Design review of the part built by this model. Coordinates are the model's own, in mm. Face numbers are marked on the shaded views. A direction names the side the tool comes from. Coordinates: 2 decimals unless noted, no trailing zeros. Write each loop counter-clockwise with the first axis right and the second up, starting at its lowest first coordinate (ties: lowest second). Pieces come first, ordered by that corner, then holes.
Q1. To check wall thickness, follow probe 1 along X at (y, z) = (6.25, 5); probe 2 along Z at (x, y) = (16.75, 2); probe 3 along Z at (x, y) = (1.25, 25). State the ranges of each line that lie inside material, in increasing order.
Q2. Add section D-D, the plane z = 59. Give the boundary of the cut face in (x, y).
Q3. Add section A-A, the plane y = 7. Give the boundary of the cut face in (x, z), plus the area to 3 significant figures.
Q4. Clearance check with flat-ended pins moving along their axes: pin 1 Ø2.5 at (x, z) = (5, 65) entering from -Y; pin 2 Ø10 at (x, z) = (9, 39) entering from -Y; pin 3 Ø6 at (x, z) = (13.5, 38.5) entering from +Y. State where each tip first meets the part, or that it passes through.
Q5. Add section C-C, the plane y = 16.5. Give the boundary of the cut face in (x, z).
Q6. Machinability: for the marked faces 1, 2 and 3, which of the approach directions +Z, -Z, +X, -X, +Y, -Y give a long, thin tool a straight path to every point of the face, cutting with its end or side? Answer none if there is none.
Q7. Add section B-B, the plane x = 9.25. Give the boundary of the cut face in (y, z), plus the area to 3 significant figures.
from build123d import *

# Parameters (mm, degrees)
ESQUISSE1_W             = 20
ESQUISSE1_H             = 31
EXTRUSION1_DEPTH        = 70
ESQUISSE2_W             = 30
ESQUISSE2_H             = 13
EXTRUSION2_DEPTH        = 80.126481029
ESQUISSE3_R             = 4.75
EXTRUSION3_DEPTH        = 75.993333037
ESQUISSE4_R             = 6
EXTRUSION4_DEPTH        = 80.126481029
ESQUISSE5_R             = 1.5
ENL_V_MAT_EXTRU_1_DEPTH = 10


with BuildPart() as part:
    # Esquisse1 → Extrusion1 (new body)
    with BuildSketch(Plane.XY):
        with Locations((10, 15.5)):
            Rectangle(ESQUISSE1_W, ESQUISSE1_H)
    extrude(amount=EXTRUSION1_DEPTH)

    # Esquisse2 → Extrusion2 (cut, through all)
    with BuildSketch(Plane(origin=(20, 0, 0), x_dir=(0, 0, -1), z_dir=(1, 0, 0))):
        with Locations((-35, 24.5)):
            Rectangle(ESQUISSE2_W, ESQUISSE2_H)
        Polygon((-45, 10), (-60, 10), (-60, 0), (-10, 0), (-10, 10), (-25, 10), (-25, 15), (-45, 15), align=None)
    extrude(amount=-EXTRUSION2_DEPTH, mode=Mode.SUBTRACT)

    # Esquisse3 → Extrusion3 (cut, through all)
    with BuildSketch(Plane(origin=(0, 18, 0), x_dir=(1, 0, 0), z_dir=(0, 1, 0))):
        with Locations(Location((10, -35, 0), (0, 0, 270))):
            Circle(ESQUISSE3_R)
    extrude(amount=-EXTRUSION3_DEPTH, mode=Mode.SUBTRACT)

    # Esquisse4 → Extrusion4 (cut, through all)
    with BuildSketch(Plane(origin=(20, 0, 0), x_dir=(0, 0, -1), z_dir=(1, 0, 0))):
        with Locations((-60, 21)):
            Circle(ESQUISSE4_R)
        with Locations((-10, 21)):
            Circle(ESQUISSE4_R)
    extrude(amount=-EXTRUSION4_DEPTH, mode=Mode.SUBTRACT)

    # Esquisse5 → Enlèv. mat.-Extru.1 (cut)
    with BuildSketch(Plane.XZ):
        with Locations(Location((5, 65, 0), (0, 0, 270))):
            Circle(ESQUISSE5_R)
        with Locations(Location((5, 5, 0), (0, 0, 270))):
            Circle(ESQUISSE5_R)
        with Locations(Location((15, 65, 0), (0, 0, 270))):
            Circle(ESQUISSE5_R)
        with Locations(Location((15, 5, 0), (0, 0, 270))):
            Circle(ESQUISSE5_R)
    extrude(amount=-ENL_V_MAT_EXTRU_1_DEPTH, mode=Mode.SUBTRACT)


solid = part.part
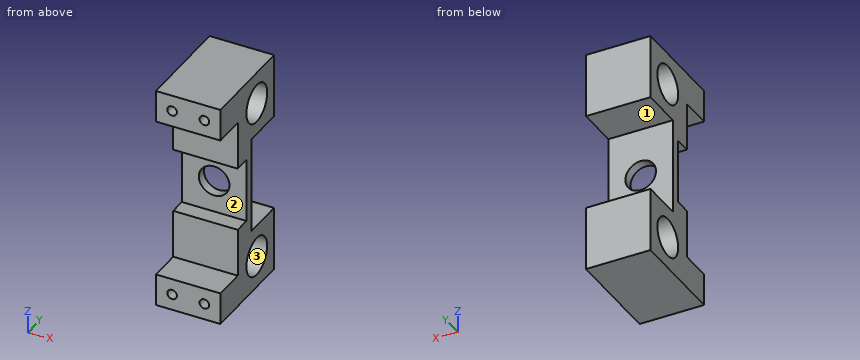
Here are the results:
1. probe 1: x = 0 to 3.5, 6.5 to 13.5, 16.5 to 20
1. probe 2: z = 0 to 10, 60 to 70
1. probe 3: z = 0 to 5.53, 14.47 to 20, 50 to 55.53, 64.47 to 70
2. outline: (0, 10) - (20, 10) - (20, 15.08) - (0, 15.08) - close; (0, 26.92) - (20, 26.92) - (20, 31) - (0, 31) - close
3. outline: (0, 0) - (20, 0) - (20, 10) - (0, 10) - close; (0, 60) - (20, 60) - (20, 70) - (0, 70) - close; hole circle Ø3 at (5, 5); hole circle Ø3 at (5, 65); hole circle Ø3 at (15, 5); hole circle Ø3 at (15, 65)
3. area: 372 mm2
4. pin 1: stops at y = 10
4. pin 2: stops at y = 15
4. pin 3: stops at y = 18
5. outline: (0, 0) - (20, 0) - (20, 6.03) - (0, 6.03) - close; (0, 13.97) - (20, 13.97) - (20, 56.03) - (0, 56.03) - close; (0, 63.97) - (20, 63.97) - (20, 70) - (0, 70) - close; hole circle Ø9.5 at (10, 35)
6. face 1: +X, -X, +Y
6. face 2: +X, -X, -Y
6. face 3: +X, -X
7. outline: (0, 0) - (31, 0) - (31, 20) - (18, 20) - (18, 30.31) - (15, 30.31) - (15, 25) - (10, 25) - (10, 10) - (0, 10) - close; (0, 60) - (10, 60) - (10, 45) - (15, 45) - (15, 39.69) - (18, 39.69) - (18, 50) - (31, 50) - (31, 70) - (0, 70) - close; hole circle Ø12 at (21, 10); hole circle Ø12 at (21, 60)
7. area: 926 mm2
